```python
from build123d import *

# Parameters (mm, degrees)
ESBO_O1_W                = 126
ESBO_O1_H                = 15
RESSALTO_EXTRUS_O1_DEPTH = 1.8
CORTE_EXTRUS_O1_DEPTH    = 64.470386796


with BuildPart() as part:
    # Esboço1 → Ressalto-extrusão1 (new body)
    with BuildSketch(Plane.XY):
        Rectangle(ESBO_O1_W, ESBO_O1_H)
    extrude(amount=RESSALTO_EXTRUS_O1_DEPTH)

    # Esboço2 → Corte-extrusão1 (cut, through all)
    with BuildSketch(Plane.XY.offset(1.8)):
        with BuildLine():
            Line((-56, 4.5), (-11, 4.5))
            ThreePointArc((-11, 4.5), (-9.5, 3), (-11, 1.5))
            Line((-11, 1.5), (-56, 1.5))
            ThreePointArc((-56, 1.5), (-57.5, 3), (-56, 4.5))
        make_face()
        with BuildLine():
            Line((-56, -4.5), (-11, -4.5))
            ThreePointArc((-11, -4.5), (-9.5, -3), (-11, -1.5))
            Line((-11, -1.5), (-56, -1.5))
            ThreePointArc((-56, -1.5), (-57.5, -3), (-56, -4.5))
        make_face()
        with BuildLine():
            Line((56, -4.5), (11, -4.5))
            ThreePointArc((11, -4.5), (9.5, -3), (11, -1.5))
            Line((11, -1.5), (56, -1.5))
            ThreePointArc((56, -1.5), (57.5, -3), (56, -4.5))
        make_face()
        with BuildLine():
            Line((56, 4.5), (11, 4.5))
            ThreePointArc((11, 4.5), (9.5, 3), (11, 1.5))
            Line((11, 1.5), (56, 1.5))
            ThreePointArc((56, 1.5), (57.5, 3), (56, 4.5))
        make_face()
    extrude(amount=-CORTE_EXTRUS_O1_DEPTH, mode=Mode.SUBTRACT)


solid = part.part
```
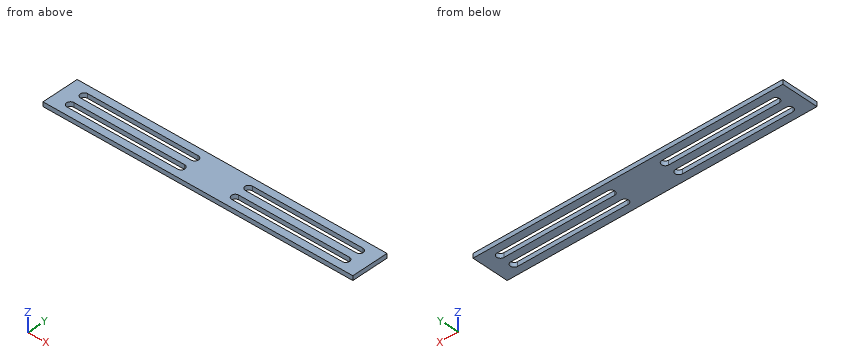
Geometry check sheet. Reference: the model listing, model coordinates, mm. Give positions to 0.01 mm unless a question says otherwise; leave off trailing zeros. Write each loop counter-clockwise with the first axis right and the second up, starting at its lowest first coordinate (ties: lowest second). Pieces come first, ordered by that corner, then holes.
1) Section check A-A, the plane x = -34. Record the boundary of the cut face in (y, z).
2) Material ranges on L1, parallel to Y at x = 17.5, z = 1.15; L2, parallel to Y at x = -10.5, z = 1.45, recorded low to high.
3) Section check B-B, the plane y = 3. Record the boundary of the cut face in (x, z), and give its area (3 significant figures).
Computed:
1. outline: (-7.5, 0) - (-4.5, 0) - (-4.5, 1.8) - (-7.5, 1.8) - close; (-1.5, 0) - (1.5, 0) - (1.5, 1.8) - (-1.5, 1.8) - close; (4.5, 0) - (7.5, 0) - (7.5, 1.8) - (4.5, 1.8) - close
2. L1: y = -7.5 to -4.5, -1.5 to 1.5, 4.5 to 7.5
2. L2: y = -7.5 to -4.41, -1.59 to 1.59, 4.41 to 7.5
3. outline: (-63, 0) - (-57.5, 0) - (-57.5, 1.8) - (-63, 1.8) - close; (-9.5, 0) - (9.5, 0) - (9.5, 1.8) - (-9.5, 1.8) - close; (57.5, 0) - (63, 0) - (63, 1.8) - (57.5, 1.8) - close
3. area: 54.0 mm2
